Read the model definition and answer for the solid it produces. Units are mm, in the model's axes. Round coordinates to 2 decimals unless told otherwise and drop trailing zeros. Loops run counter-clockwise (first coordinate to the right, second up) from the corner with the lowest first, then second, coordinate; pieces in that order, holes last. Notation, with made-up numbers: (20.25, 74.25) -> (49.25, 74.25) arc R9 ccw to (49.25, 90.25) -> close; hole circle Ø2 at (32, 21.5). An arc over 180 degrees is marked (long way). Put each result on its own line as item: value.
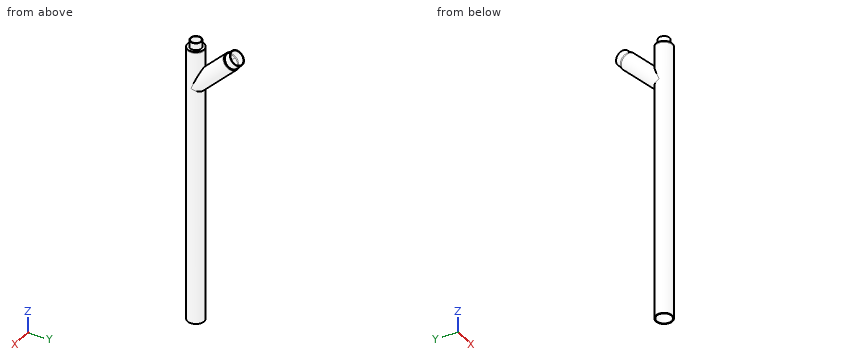
from build123d import *
from build123d import SkipClean  # not in build123d's __all__

# Parameters (mm, degrees)
F3_R      = 30
F3_R_2    = 27
F5_R      = 30
F5_R_2    = 27
F7_R      = 27
F8_DEPTH  = 1000.001
F9_R      = 27
F10_REACH = 885.9968684831
F11_R     = 30
F11_R_2   = 27
F12_DEPTH = 5
F13_R     = 20
F13_R_2   = 18
F14_DEPTH = 25
F15_R     = 18
F16_DEPTH = 25
F17_R     = 30
F17_R_2   = 27
F18_DEPTH = 5
F19_R     = 27
F19_R_2   = 25
F20_DEPTH = 25
F21_R     = 25
F22_DEPTH = 25


with BuildPart() as f4:
    # F4: sweep along a path in F0
    with BuildLine(Plane.YZ) as f4_path:
        Line((0, -487.5), (0, 380))
        Line((0, 380), (123.7436867076, 503.7436867076))
    # F3 (on plane+point) → F4 (sweep)
    with BuildSketch(Plane.XY.offset(-487.5)):
        Circle(F3_R)
        Circle(F3_R_2, mode=Mode.SUBTRACT)
    sweep(path=f4_path.line, transition=Transition.RIGHT)

    # F6: sweep along a path in F0
    with BuildLine(Plane.YZ) as f6_path:
        Line((0, 512.5), (0, 380))
    # F5 (on plane+point) → F6 (sweep)
    with BuildSketch(Plane.XY.offset(380)):
        Circle(F5_R)
        Circle(F5_R_2, mode=Mode.SUBTRACT)
    sweep(path=f6_path.line)

    # F7 (on face) → F8 (cut, through all)
    with BuildSketch(Plane.XY.offset(512.5)):
        Circle(F7_R)
    extrude(amount=-F8_DEPTH, mode=Mode.SUBTRACT)

    f10_end = f4.faces().sort_by_distance((-27, 0, 12.5))[0]
    # F9 (on face) → F10 (cut, up to a face of the model that its end follows)
    with BuildSketch(Plane(origin=(0, 313.7436867076, 313.7436867076), x_dir=(-1, 0, 0), z_dir=(0, 0.7071067812, 0.7071067812))):
        with Locations((0, 268.7005768509)):
            Circle(F9_R)
    f10_long = extrude(amount=-F10_REACH, mode=Mode.PRIVATE)
    add(split(f10_long, bisect_by=f10_end, keep=Keep.TOP, mode=Mode.PRIVATE), mode=Mode.SUBTRACT)

    # F11 (on face) → F12 (join)
    with BuildSketch(Plane.XY.offset(512.5)):
        Circle(F11_R)
        Circle(F11_R_2, mode=Mode.SUBTRACT)
        Circle(F11_R_2)
    with SkipClean():  # cleaning this boolean's faces spoils the solid; the shape is the same uncleaned
        extrude(amount=F12_DEPTH)

    # F13 (on face) → F14 (join)
    with BuildSketch(Plane.XY.offset(517.5)):
        Circle(F13_R)
        Circle(F13_R_2, mode=Mode.SUBTRACT)
    extrude(amount=F14_DEPTH)

    # F15 (on face) → F16 (cut)
    with BuildSketch(Plane.XY.offset(517.5)):
        Circle(F15_R)
    extrude(amount=-F16_DEPTH, mode=Mode.SUBTRACT)

    # F17 (on face) → F18 (join)
    with BuildSketch(Plane(origin=(0, 313.7436867076, 313.7436867076), x_dir=(-1, 0, 0), z_dir=(0, 0.7071067812, 0.7071067812))):
        with Locations((0, 268.7005768509)):
            Circle(F17_R)
        with Locations((0, 268.7005768509)):
            Circle(F17_R_2, mode=Mode.SUBTRACT)
        with Locations((0, 268.7005768509)):
            Circle(F17_R_2)
    extrude(amount=F18_DEPTH)

    # F19 (on face) → F20 (join)
    with BuildSketch(Plane(origin=(0, 317.2792206136, 317.2792206136), x_dir=(-1, 0, 0), z_dir=(0, 0.7071067812, 0.7071067812))):
        with Locations((0, 268.7005768509)):
            Circle(F19_R)
        with Locations((0, 268.7005768509)):
            Circle(F19_R_2, mode=Mode.SUBTRACT)
    extrude(amount=F20_DEPTH)

    # F21 (on face) → F22 (cut)
    with BuildSketch(Plane(origin=(0, 317.2792206136, 317.2792206136), x_dir=(-1, 0, 0), z_dir=(0, 0.7071067812, 0.7071067812))):
        with Locations((0, 268.7005768509)):
            Circle(F21_R)
    extrude(amount=-F22_DEPTH, mode=Mode.SUBTRACT)


solid = f4.part
Item 1: The part is cut by section A-A (x = 0). State how many separate pieces and enclosed holes the cut face has, then the cut area to 3 significant figures.
Derived:
separate pieces: 3
enclosed holes: 0
area: 6,940 mm^2
Item 2: The part is cut by section C-C (z = 305). Determine the outline of the cut face in (x, y).
Derived:
outline: circle Ø60 at (0, 0); hole circle Ø54 at (0, 0)
Item 3: Find the intervals of material crossed by line 1 along Y through (x, z) = (2.5, 480.5); line 2 along Y through (x, z) = (0, -30); line 3 along Z through (x, y) = (21, -12.5), in increasing order.
Derived:
line 1: y = -29.9 to -26.88, 26.88 to 29.9, 58.22 to 62.48, 138.52 to 142.78
line 2: y = -30 to -27, 27 to 30
line 3: z = 512.5 to 517.5
Item 4: Flat-ended cylindrical pins translate along their axes: pin 1 Ø5 at (x, z) = (-21.5, -181.5) entering from +Y; pin 2 Ø4 at (x, y) = (17, 37) entering from -Z; pin 3 Ø5 at (x, y) = (-4.5, 44.5) entering from -Z; pin 4 Ø16 at (x, y) = (4.5, 3.5) entering from -Z. Find the tip coordinate at first contact, or state that the pin passes through.
Derived:
pin 1: stops at y = 23.22
pin 2: stops at z = 379.33
pin 3: stops at z = 380
pin 4: passes through
Item 5: The part is cut by section B-B (y = -9). Determine the outline of the cut face in (x, z).
Derived:
outline: (-28.62, -487.5) -> (-25.46, -487.5) -> (-25.46, 512.5) -> (-15.59, 512.5) -> (-15.59, 542.5) -> (-17.86, 542.5) -> (-17.86, 517.5) -> (-28.62, 517.5) -> close; (15.59, 512.5) -> (25.46, 512.5) -> (25.46, -487.5) -> (28.62, -487.5) -> (28.62, 517.5) -> (17.86, 517.5) -> (17.86, 542.5) -> (15.59, 542.5) -> close
